```python
from build123d import *

# Parameters (mm, degrees)
F1_DEPTH  = 13
F4_DEPTH  = 13.001
F5_R      = 0.49999
F6_R      = 1
F7_R      = 5
F8_R      = 1
F9_R      = 0.5
F10_R     = 1
F11_R     = 1.75
F12_DEPTH = 15.6999998824


# Not quite as in the source:
# - a fillet or chamfer is up to 0.001 mm smaller than in the source, because OpenCascade refuses the exact size


with BuildPart() as f1:
    # F0 (on Top) → F1 (new body)
    with BuildSketch(Plane.XY):
        with BuildLine():
            ThreePointArc((-14.5, 1), (-14.2071067812, 0.2928932188), (-13.5, 0))
            Line((-13.5, 0), (-5.6426405208, 0))
            Line((-5.6426405208, 0), (-13.2228966419, -7.5802561211))
            Line((-13.2228966419, -7.5802561211), (0, -20.803152763))
            Line((0, -20.803152763), (13.2228966419, -7.5802561211))
            Line((13.2228966419, -7.5802561211), (5.6426405208, 0))
            Line((5.6426405208, 0), (13.5, 0))
            ThreePointArc((13.5, 0), (14.2071067812, 0.2928932188), (14.5, 1))
            Line((14.5, 1), (14.5, 9.5887489808))
            ThreePointArc((14.5, 9.5887489808), (12.0898455808, 8.3182698074), (11.05, 5.8))
            Line((11.05, 5.8), (12.8, 5.8))
            Line((12.8, 5.8), (12.8, 2.8))
            Line((12.8, 2.8), (9.55, 2.8))
            ThreePointArc((9.55, 2.8), (8.8, 3.55), (8.05, 2.8))
            Line((8.05, 2.8), (-8.05, 2.8))
            ThreePointArc((-8.05, 2.8), (-8.8, 3.55), (-9.55, 2.8))
            Line((-9.55, 2.8), (-12.8, 2.8))
            Line((-12.8, 2.8), (-12.8, 5.8))
            Line((-12.8, 5.8), (-11.05, 5.8))
            ThreePointArc((-11.05, 5.8), (-12.0898455808, 8.3182698074), (-14.5, 9.5887489808))
            Line((-14.5, 9.5887489808), (-14.5, 1))
        make_face()
        with BuildLine():
            Line((-8.6267027305, -7.2267027305), (-0.3535533906, 1.0464466094))
            ThreePointArc((-0.3535533906, 1.0464466094), (0, 1.9), (0.3535533906, 1.0464466094))
            Line((0.3535533906, 1.0464466094), (8.6267027305, -7.2267027305))
            ThreePointArc((8.6267027305, -7.2267027305), (9.4802561211, -7.5802561211), (8.6267027305, -7.9338095117))
            Line((8.6267027305, -7.9338095117), (0.3535533906, -16.2069588515))
            ThreePointArc((0.3535533906, -16.2069588515), (0, -17.0605122421), (-0.3535533906, -16.2069588515))
            Line((-0.3535533906, -16.2069588515), (-8.6267027305, -7.9338095117))
            ThreePointArc((-8.6267027305, -7.9338095117), (-9.4802561211, -7.5802561211), (-8.6267027305, -7.2267027305))
        make_face(mode=Mode.SUBTRACT)
    extrude(amount=F1_DEPTH)

    # F3 (on face) → F4 (cut, through all)
    with BuildSketch(Plane.XY.offset(13)):
        with BuildLine():
            ThreePointArc((-14.5, 5.8), (-14.0485078359, 7.3827532374), (-14.5, 8.9655064748))
            Line((-14.5, 8.9655064748), (-14.5, 5.8))
        make_face()
        with BuildLine():
            Line((14.5, 5.8), (14.5, 8.9655064748))
            ThreePointArc((14.5, 8.9655064748), (14.0485078359, 7.3827532374), (14.5, 5.8))
        make_face()
    extrude(amount=-F4_DEPTH, mode=Mode.SUBTRACT)

    # F5 (radius 0.5 in the source; OpenCascade refuses exactly that, so slightly less here)
    f5_edges = [f1.edges().sort_by_distance(p)[0] for p in [
        (-14.5, 9.588749, 6.5),
        (14.5, 9.588749, 6.5),
    ]]
    fillet(f5_edges, radius=F5_R)

    # F6
    f6_edges = [f1.edges().sort_by_distance(p)[0] for p in [
        (-5.642641, 0, 6.5),
        (5.642641, 0, 6.5),
    ]]
    fillet(f6_edges, radius=F6_R)

    # F7
    f7_edges = [f1.edges().sort_by_distance(p)[0] for p in [
        (-13.222897, -7.580256, 6.5),
        (0, -20.803153, 6.5),
        (13.222897, -7.580256, 6.5),
    ]]
    fillet(f7_edges, radius=F7_R)

    # F8
    f8_edges = [f1.edges().sort_by_distance(p)[0] for p in [
        (-6.611448, -14.191704, 13),
        (-6.611448, -14.191704, 0),
    ]]
    fillet(f8_edges, radius=F8_R)

    # F9
    f9_edges = [f1.edges().sort_by_distance(p)[0] for p in [
        (-11.05, 5.8, 6.5),
        (11.05, 5.8, 6.5),
    ]]
    fillet(f9_edges, radius=F9_R)

    # F10
    f10_edges = [f1.edges().sort_by_distance(p)[0] for p in [
        (-0.353553, 1.046447, 6.5),
        (0.353553, 1.046447, 6.5),
        (-8.626703, -7.226703, 6.5),
        (-8.626703, -7.93381, 6.5),
        (-0.353553, -16.206959, 6.5),
        (0.353553, -16.206959, 6.5),
        (8.626703, -7.226703, 6.5),
        (8.626703, -7.93381, 6.5),
    ]]
    fillet(f10_edges, radius=F10_R)

    # F11 (on face) → F12 (cut, through all)
    with BuildSketch(Plane(origin=(10.4015763815, -10.4015763815, 0), x_dir=(0.7071067812, 0.7071067812, 0), z_dir=(0.7071067812, -0.7071067812, 0))):
        with Locations((-5.3600505063, 6.5)):
            Circle(F11_R)
    extrude(amount=-F12_DEPTH, mode=Mode.SUBTRACT)


solid = f1.part
```
The model under review builds one solid part; all positions refer to its coordinate system, in mm. A direction names the side the tool comes from. Round coordinates to 2 decimals unless told otherwise and drop trailing zeros. Loops run counter-clockwise (first coordinate to the right, second up) from the corner with the lowest first, then second, coordinate; pieces in that order, holes last. Notation, with made-up numbers: M -17,78 L 4,78 A33 ccw 4,109 Z; hole C 12.25,63.25 d10. An arc over 180 degrees is marked long. Answer as a JSON object with one key per item and string values.
(1) Draft analysis for pull direction X (two halves, no side actions). For faces 4 (the flat face through (11, 0, 6)), 5 (the flat face through (12, 5.8, 6)), 6 (the cylindrical face through (-8.322, -3.105, 0.285)), state which applies: released by +X, released by -X, zero draft, split by the parting line, or undercut.
Resolved:
{"face 4": "zero draft", "face 5": "undercut", "face 6": "released by -X"}
(2) Clearance check with flat-ended pins moving along their axes: P1, Ø0.6, axis at x = 12.5, z = 6.5, coming from the -Y side; P2, Ø2.5, axis at x = -12, z = 5.5, coming from the -Y side; P3, Ø1.5, axis at x = -10, z = 10, coming from the -Y side; P4, Ø6, axis at x = -0.5, y = -11.5, coming from the +Z side. State where each tip first meets the part, or that it passes through.
Resolved:
{"P1": "y = 0", "P2": "y = -9.54", "P3": "y = -11.55", "P4": "through"}
(3) Tool access review of faces 1 (the cylindrical face through (-6.4, -14, 12.7)), 2 (the flat face through (4.4, -3, 6.4)), 3 (the cylindrical face through (12.09, 8.32, 6.41)): name each direction out of +Z, -Z, +X, -X, +Y, -Y from which nothing blocks a thin tool from reaching the whole face with its end or side.
Resolved:
{"face 1": "+Z, -X, -Y", "face 2": "+Z, -Z", "face 3": "+Z, -Z, +Y"}
(4) To check wall thickness, follow line 1 along X through (y, z) = (-7.5, 6.75); line 2 along Y through (x, z) = (9, 7.75); line 3 along Y through (x, z) = (7.25, 1). State the ranges of each line that lie inside material, in increasing order.
Resolved:
{"line 1": "-11.15 to -9.47, 9.47 to 11.15", "line 2": "-11.8 to -8.08, -7.08 to -3.36, 0 to 3.52", "line 3": "-13.55 to -9.31, -5.85 to -1.59, -0.41 to 2.8"}
(5) Take a section at B-B on y = 7.5. Give the boundary of the cut face in (x, z), and give its area (3 significant figures).
Resolved:
{"outline": "M -14.05,0.17 A1 ccw -13.5,0 L -11.51,0 L -11.51,13 L -13.5,13 A1 ccw -14.05,12.83 Z; M 11.51,0 L 13.5,0 A1 ccw 14.05,0.17 L 14.05,12.83 A1 ccw 13.5,13 L 11.51,13 Z", "area": "65.8 mm²"}
(6) Take a section at A-A on x = 0. Give the boundary of the cut face in (y, z), and give its area (3 significant figures).
Resolved:
{"outline": "M -18.73,1 A1 ccw -17.73,0 L -17.06,0 L -17.06,13 L -17.73,13 A1 ccw -18.73,12 Z; M 1.9,0 L 2.8,0 L 2.8,13 L 1.9,13 Z", "area": "33.0 mm²"}
